Work out the finished part from the listing and answer in its coordinate system (mm). Face numbers are marked on the shaded views. A direction names the side the tool comes from. Round coordinates to 2 decimals unless told otherwise and drop trailing zeros. Write each loop counter-clockwise with the first axis right and the second up, starting at its lowest first coordinate (ties: lowest second). Pieces come first, ordered by that corner, then holes.
Autodesk Fusion 360 part; units mm, degrees
sketch "Sketch6" plane through (0, 0, 0) normal (0, 0, 1) x (1, 0, 0)
  line L0 (0, 0) -> (24, 0)
  line L1 (24, 0) -> (24, 9)
  line L2 (24, 9) -> (0, 9)
  line L3 (0, 9) -> (0, 0)
  line L4 (24, 9) -> (26.5, 9) construction
  line L5 (26.5, 9) -> (26.5, 11.5) construction
  line L6 (0, 0) -> (-2.5, 0) construction
  line L7 (-2.5, 0) -> (-2.5, -2.5) construction
  line L8 (26.5, 11.5) -> (-2.5, 11.5)
  line L9 (-2.5, 11.5) -> (-2.5, -2.5)
  line L10 (-2.5, -2.5) -> (26.5, -2.5)
  line L11 (26.5, -2.5) -> (26.5, 11.5)
  dimension "d28" = 24
  dimension "d29" = 9
  dimension "d32" = 2.5
  dimension "d33" = 2.5
  dimension "d34" = 2.5
  dimension "d35" = 2.5
extrude "Extrude8" add sketch "Sketch6" along normal blind 3.5 contours L0 L1 L2 L3
sketch "Sketch7" plane through (0, 0, 3.5) normal (0, 0, 1) x (-1, 0, 0)
  line L0 (0, -9) -> (0, 0)
  line L1 (0, 0) -> (-24, 0)
  line L2 (-24, 0) -> (-24, -9)
  line L3 (-24, -9) -> (0, -9)
  line L4 (-12, -9) -> (-10, -9)
  line L5 (-10, -9) -> (-10, 0)
  line L6 (-10, 0) -> (-12, 0)
  line L7 (-12, 0) -> (-12, -9)
extrude "Extrude9" add sketch "Sketch7" along normal blind 2 contours L1 L3 L4 L5 L6 L7
sketch "Sketch8" plane through (0, 0, 0) normal (0, 0, -1) x (1, 0, 0)
  line L0 (0, 0) -> (0, -9)
  line L1 (0, -9) -> (24, -9)
  line L2 (24, -9) -> (24, 0)
  line L3 (24, 0) -> (0, 0)
  line L4 (12, 0) -> (12, -9) construction
  line L5 (15.4, -7.9) -> (8.6, -7.9)
  line L6 (8.6, -7.9) -> (8.6, -1.1)
  line L7 (8.6, -1.1) -> (15.4, -1.1)
  line L8 (15.4, -1.1) -> (15.4, -7.9)
  line L9 (15.4, -7.9) -> (8.6, -1.1) construction
  line L10 (8.6, -7.9) -> (15.4, -1.1) construction
  point P0 (12, -4.5)
  dimension "d39" = 6.8
  dimension "d40" = 6.8
extrude "Extrude10" cut sketch "Sketch8" against normal blind 3 contours L5 L6 L7 L8
extrude "Extrude13" add sketch "Sketch6" along normal blind 11.5
sketch "Sketch10" plane through (0, 0, 11.5) normal (0, 0, 1) x (-1, 0, 0)
  line L0 (0, 0) -> (0, -9)
  line L1 (0, -9) -> (-24, -9)
  line L2 (-24, -9) -> (-24, 0)
  line L3 (-24, 0) -> (0, 0)
  line L4 (-26.5, 2.5) -> (-26.5, -11.5)
  line L5 (-26.5, -11.5) -> (2.5, -11.5)
  line L6 (2.5, -11.5) -> (2.5, 2.5)
  line L7 (2.5, 2.5) -> (-26.5, 2.5)
  line L8 (-24, 0) -> (-26.5, 0)
  line L9 (-26.5, 0) -> (-26.5, -3)
  line L10 (-26.5, -3) -> (-24, -3)
  line L11 (-24, -3) -> (-24, 0)
  line L12 (-24, -9) -> (-26.5, -9)
  line L13 (-26.5, -9) -> (-26.5, -6)
  line L14 (-26.5, -6) -> (-24, -6)
  line L15 (-24, -6) -> (-24, -9)
  dimension "d50" = 3
  dimension "d51" = 3
extrude "Extrude14" cut sketch "Sketch10" against normal blind 4 contours L2 L4 L8 L9 L10 L11 | L2 L4 L12 L13 L14 L15
sketch "Sketch11" plane through (0, 11.5, 0) normal (0, 1, 0) x (-1, 0, 0)
  line L0 (-26.5, 0) -> (2.5, 0)
  line L1 (2.5, 0) -> (2.5, 11.5)
  line L2 (2.5, 11.5) -> (-26.5, 11.5)
  line L3 (-26.5, 11.5) -> (-26.5, 0)
  line L4 (-12, 11.5) -> (-7, 11.5) construction
  line L5 (-7, 11.5) -> (-17, 11.5)
  line L6 (-17, 11.5) -> (-17, 8.5)
  line L7 (-17, 8.5) -> (-7, 8.5)
  line L8 (-7, 8.5) -> (-7, 11.5)
  dimension "d54" = 5
  dimension "d55" = 10
  dimension "d56" = 3
extrude "Extrude15" add sketch "Sketch11" along normal blind 9 contours L2 L5 L6 L7 L8
sketch "Sketch12" plane through (0, -2.5, 0) normal (0, -1, 0) x (1, 0, 0)
  line L0 (-2.5, 0) -> (26.5, 0)
  line L1 (26.5, 0) -> (26.5, 11.5)
  line L2 (26.5, 11.5) -> (-2.5, 11.5)
  line L3 (-2.5, 11.5) -> (-2.5, 0)
  line L4 (12, 11.5) -> (17, 11.5) construction
  line L5 (17, 11.5) -> (7, 11.5)
  line L6 (7, 11.5) -> (7, 8.5)
  line L7 (7, 8.5) -> (17, 8.5)
  line L8 (17, 8.5) -> (17, 11.5)
  dimension "d59" = 5
  dimension "d60" = 10
  dimension "d61" = 3
extrude "Extrude16" add sketch "Sketch12" along normal blind 9 contours L2 L5 L6 L7 L8
fillet "Fillet1" radius 5.5 2 edges at (12, -2.5, 8.5) (12, 11.5, 8.5)
fillet "Fillet2" radius 3 4 edges at (17, 20.5, 10) (7, 20.5, 10) (17, -11.5, 10) (7, -11.5, 10)
fillet "Fillet3" radius 2 4 edges at (-2.5, 11.5, 5.75) (-2.5, -2.5, 5.75) (26.5, 11.5, 5.75) (26.5, -2.5, 5.75)
fillet "Fillet4" radius 2 4 edges at (7, -2.5, 7.25) (17, -2.5, 7.25) (17, 11.5, 7.25) (7, 11.5, 7.25)
sketch "Sketch13" plane through (0, 0, 11.5) normal (0, 0, 1) x (-1, 0, 0)
  arc A0 (-24.5, 2.5) -> (-26.5, 0.5) centre (-24.5, 0.5) ccw
  line L0 (-26.5, 0.5) -> (-26.5, 0)
  line L1 (-26.5, 0) -> (0, 0)
  line L2 (0, 0) -> (0, -9)
  line L3 (0, -9) -> (-26.5, -9)
  line L4 (-26.5, -9) -> (-26.5, -9.5)
  arc A1 (-26.5, -9.5) -> (-24.5, -11.5) centre (-24.5, -9.5) ccw
  line L5 (-24.5, -11.5) -> (-19, -11.5)
  arc A2 (-17, -13.5) -> (-19, -11.5) centre (-19, -13.5) ccw
  line L6 (-17, -13.5) -> (-17, -17.5)
  arc A3 (-17, -17.5) -> (-14, -20.5) centre (-14, -17.5) ccw
  line L7 (-14, -20.5) -> (-10, -20.5)
  arc A4 (-10, -20.5) -> (-7, -17.5) centre (-10, -17.5) ccw
  line L8 (-7, -17.5) -> (-7, -13.5)
  arc A5 (-5, -11.5) -> (-7, -13.5) centre (-5, -13.5) ccw
  line L9 (-5, -11.5) -> (0.5, -11.5)
  arc A6 (0.5, -11.5) -> (2.5, -9.5) centre (0.5, -9.5) ccw
  line L10 (2.5, -9.5) -> (2.5, 0.5)
  arc A7 (2.5, 0.5) -> (0.5, 2.5) centre (0.5, 0.5) ccw
  line L11 (0.5, 2.5) -> (-5, 2.5)
  arc A8 (-7, 4.5) -> (-5, 2.5) centre (-5, 4.5) ccw
  line L12 (-7, 4.5) -> (-7, 8.5)
  arc A9 (-7, 8.5) -> (-10, 11.5) centre (-10, 8.5) ccw
  line L13 (-10, 11.5) -> (-14, 11.5)
  arc A10 (-14, 11.5) -> (-17, 8.5) centre (-14, 8.5) ccw
  line L14 (-17, 8.5) -> (-17, 4.5)
  arc A11 (-19, 2.5) -> (-17, 4.5) centre (-19, 4.5) ccw
  line L15 (-19, 2.5) -> (-24.5, 2.5)
  line L16 (-12, -20.5) -> (-12, -16) construction
  line L17 (-12, 11.5) -> (-12, 7) construction
  circle A12 centre (-12, -16) radius 0.75
  circle A13 centre (-12, 7) radius 0.75
  dimension "d72" = 4.5
  dimension "d73" = 1.5
  dimension "d74" = 1.5
extrude "Extrude17" cut sketch "Sketch13" against normal blind 5 contours A12 | A13
sketch "Sketch14" plane through (0, 0, 3) normal (0, 0, -1) x (1, 0, 0)
  line L0 (15.4, -1.1) -> (8.6, -1.1)
  line L1 (8.6, -1.1) -> (8.6, -7.9)
  line L2 (8.6, -7.9) -> (15.4, -7.9)
  line L3 (15.4, -7.9) -> (15.4, -1.1)
  line L4 (12, -1.1) -> (12.5, -1.1)
  line L5 (12.5, -1.1) -> (11.5, -1.1)
  line L6 (11.5, -1.1) -> (11.5, -2.3)
  line L7 (11.5, -2.3) -> (12.5, -2.3)
  line L8 (12.5, -2.3) -> (12.5, -1.1)
  line L9 (12, -7.9) -> (11.5, -7.9)
  line L10 (11.5, -7.9) -> (12.5, -7.9)
  line L11 (12.5, -7.9) -> (12.5, -6.7)
  line L12 (12.5, -6.7) -> (11.5, -6.7)
  line L13 (11.5, -6.7) -> (11.5, -7.9)
  dimension "d77" = 0.5
  dimension "d78" = 1
  dimension "d79" = 1.2
  dimension "d80" = 0.5
  dimension "d81" = 1
  dimension "d82" = 1.2
extrude "Extrude18" cut sketch "Sketch14" against normal up to surface (2.5 mm away) contours L0 L4 L5 L6 L7 L8 | L2 L9 L10 L11 L12 L13
fillet "Fillet5" radius 2 8 edges at (12, -2.5, 0) (25.9142, -1.9142, 0) (26.5, 4.5, 0) (25.9142, 10.9142, 0) (12, 11.5, 0) (-1.9142, 10.9142, 0) (-2.5, 4.5, 0) (-1.9142, -1.9142, 0)
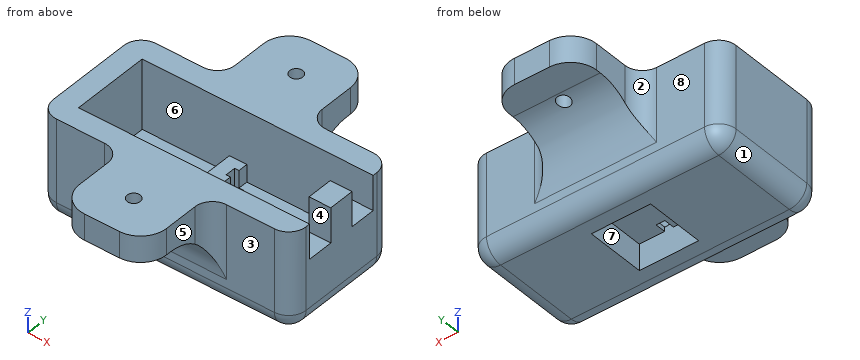
Q1. A tool of negligible diameter and unlimited length cuts with its end or side. For the marked faces 5, 6, 7 and 8, from which of +Z, -Z, +X, -X, +Y, -Y can it reach the whole face along a straight path? Write none if from no direction.
Q2. Find section D-D (x = 16.5). Determine the outline of the cut face in (y, z), plus the area to 3 significant figures.
Q3. Find section A-A (z = 10). Count the separate pieces of the cut face and the enclosed holes in it, plus the area to 3 significant figures.
Q4. Find section C-C (z = 6). Determine the outline of the cut face in (x, y), plus the area to 3 significant figures.
Q5. The mould has two halves that part along Y. Classify the marked faces 1, 2, 3 and 4: +Y half, -Y half, draft (parallel to the pull), parting line (faces both ways), or undercut.
Q6. Find the intervals of material crossed by L1, parallel to Y at x = 12, z = 9.25; L2, parallel to Y at x = 1, z = 5.5; L3, parallel to X at y = -7, z = 9.25, in increasing order.
Q7. Given pin 1 (3 mm diameter, centred on x = 10.5, z = 3, fed in from +Y); pin 2 (3 mm diameter, centred on y = -6.5, z = 9, fed in from -X); pin 3 (3 mm diameter, centred on x = 15, z = 5, fed in from -Y), each flat-ended and moving along its own axis, determine where each tip first touches the part or whether it passes through.
Q8. Find section B-B (y = -7). Determine the outline of the cut face in (x, z), plus the area to 3 significant figures.
Report:
1. face 5: +Z, -Z, +X, -Y
1. face 6: +Z
1. face 7: -Z
1. face 8: -Z, +Y
2. outline: (-10.16, 8.5) - (-8, 8.5) arc R5.5 cw to (-2.5, 3) - (-2.5, 2) arc R2 ccw to (-0.5, 0) - (9.5, 0) arc R2 ccw to (11.5, 2) - (11.5, 3) arc R5.5 cw to (17, 8.5) - (19.16, 8.5) - (19.16, 11.5) - (9, 11.5) - (9, 3.5) - (0, 3.5) - (0, 11.5) - (-10.16, 11.5) - close
2. area: 146 mm2
3. separate pieces: 2
3. enclosed holes: 2
3. area: 344 mm2
4. outline: (-2.5, -0.5) arc R2 ccw to (-0.5, -2.5) - (5, -2.5) arc R2 cw to (6.66, -3.39) - (17.34, -3.39) arc R2 cw to (19, -2.5) - (24.5, -2.5) arc R2 ccw to (26.5, -0.5) - (26.5, 9.5) arc R2 ccw to (24.5, 11.5) - (19, 11.5) arc R2 cw to (17.34, 12.39) - (6.66, 12.39) arc R2 cw to (5, 11.5) - (-0.5, 11.5) arc R2 ccw to (-2.5, 9.5) - close; hole (0, 0) - (24, 0) - (24, 9) - (0, 9) - close
4. area: 207 mm2
5. face 1: draft
5. face 2: +Y half
5. face 3: -Y half
5. face 4: undercut
6. L1: y = -11.5 to -7.75, -6.25 to 0, 9 to 15.25, 16.75 to 20.5
6. L2: y = -2.5 to 0, 9 to 11.5
6. L3: x = 7 to 11.25, 12.75 to 17
7. pin 1: stops at y = 11.71
7. pin 2: stops at x = 7
7. pin 3: stops at y = -3.76
8. outline: (7, 8.41) - (11.25, 8.41) - (11.25, 11.5) - (7, 11.5) - close; (12.75, 8.41) - (17, 8.41) - (17, 11.5) - (12.75, 11.5) - close
8. area: 26.3 mm2
